Verification items for the finished model (mm, model axes). Face numbers are marked on the shaded views. A direction names the side the tool comes from. Give positions to 0.01 mm unless a question says otherwise; leave off trailing zeros. Order: outer loops, then holes, each group sorted by start corner. A loop starts at its lowest first (then second) coordinate and runs counter-clockwise, first axis right, second up.
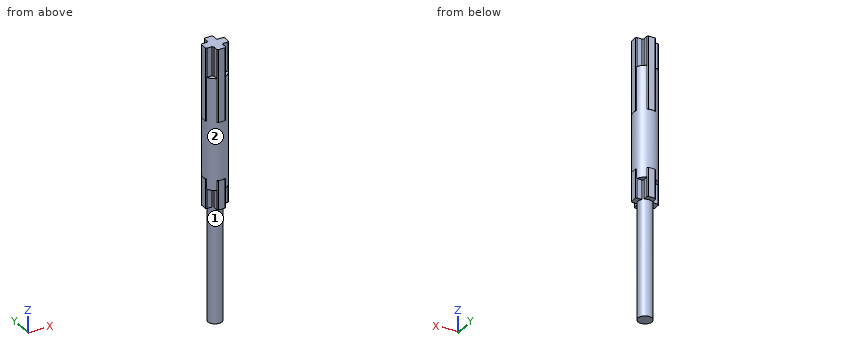
Autodesk Inventor part; units mm, degrees
ref_plane "Plano de trabajo1" through (0, -3.8636, 23) normal (0, 0, -1) x (-1, 0, 0)
ref_plane "Plano de trabajo2" through (0, 0, 0) normal (0, 0, 1) x (1, 0, 0)
ref_plane "YZ Plane" through (0, 0, 0) normal (1, 0, 0) x (0, 1, 0)
sketch "Boceto2" plane through (0, 0, 0) normal (0, 0, 1) x (1, 0, 0)
  line L0 (0.9, -6.2636) -> (-0.9, -6.2636)
  line L1 (-0.9, -6.2636) -> (-0.9, -1.4636)
  line L2 (-0.9, -1.4636) -> (0.9, -1.4636)
  line L3 (0.9, -1.4636) -> (0.9, -6.2636)
  line L4 (0.9, -6.2636) -> (-0.9, -1.4636) construction
  line L5 (-0.9, -6.2636) -> (0.9, -1.4636) construction
  line L6 (-2.4, -4.7636) -> (2.4, -4.7636)
  line L7 (2.4, -4.7636) -> (2.4, -2.9636)
  line L8 (2.4, -2.9636) -> (-2.4, -2.9636)
  line L9 (-2.4, -2.9636) -> (-2.4, -4.7636)
  line L10 (-2.4, -4.7636) -> (2.4, -2.9636) construction
  line L11 (2.4, -4.7636) -> (-2.4, -2.9636) construction
  circle A0 centre (0, -3.8636) radius 1.45
  point P0 (0, 0)
  point P1 (1.1369, -2.9636)
  point P2 (0.9, -2.7267)
  point P3 (-0.9, -2.7267)
  point P4 (-1.1369, -2.9636)
  point P5 (-1.1369, -4.7636)
  point P6 (-0.9, -5.0005)
  point P7 (0.9, -5.0005)
  point P8 (1.1369, -4.7636)
  dimension "d0" = 4.8
  dimension "d1" = 1.8
  dimension "d2" = 1.8
  dimension "d3" = 4.8
  dimension "d4" = 2.9
extrude "Extrusión1" add sketch "Boceto2" along normal blind 2 and the other way blind 4
sketch "Boceto3" plane through (0, 0, 2) normal (0, 0, 1) x (1, 0, 0)
  arc A0 (-0.9, -2.7267) -> (-1.1369, -2.9636) centre (0, -3.8636) ccw construction
  circle A1 centre (0, -3.8636) radius 1.45
  arc A2 (1.1369, -2.9636) -> (0.9, -2.7267) centre (0, -3.8636) ccw construction
  point P0 (0, 0)
  point P1 (1.0253, -2.8383)
extrude "Extrusión2" add sketch "Boceto3" along normal blind 12 and the other way blind 30
sketch "Boceto4" plane through (0, -3.8636, 14) normal (0, 0, 1) x (1, 0, 0)
  circle A0 centre (0, 0) radius 1.45 construction
  circle A1 centre (0, 0) radius 1.45
  line L0 (-0.9, 2.4) -> (0.9, 2.4) construction
  line L1 (0.9, -2.4) -> (-0.9, -2.4)
  line L2 (-0.9, -2.4) -> (-0.9, 2.4)
  line L3 (-0.9, 2.4) -> (0.9, 2.4)
  line L4 (0.9, 2.4) -> (0.9, -2.4)
  line L5 (0.9, -2.4) -> (-0.9, 2.4) construction
  line L6 (-0.9, -2.4) -> (0.9, 2.4) construction
  line L7 (2.4, 0.9) -> (-2.4, 0.9)
  line L8 (-2.4, 0.9) -> (-2.4, -0.9)
  line L9 (-2.4, -0.9) -> (2.4, -0.9)
  line L10 (2.4, -0.9) -> (2.4, 0.9)
  line L11 (2.4, 0.9) -> (-2.4, -0.9) construction
  line L12 (-2.4, 0.9) -> (2.4, -0.9) construction
  point P0 (1.1369, 0.9)
  point P1 (0.9, 1.1369)
  point P2 (-0.9, 1.1369)
  point P3 (-1.1369, 0.9)
  point P4 (-1.1369, -0.9)
  point P5 (-0.9, -1.1369)
  point P6 (0.9, -1.1369)
  point P7 (1.1369, -0.9)
extrude "Extrusión3" add sketch "Boceto4" along normal blind 15
chamfer "Chaflán1" distance 0.2 angle 45 16 edges at (0.9, -1.4636, -1) (-0.9, -1.4636, -1) (-2.4, -2.9636, -1) (-2.4, -4.7636, -1) (-0.9, -6.2636, -1) (0.9, -6.2636, -1) (2.4, -4.7636, -1) (2.4, -2.9636, -1) (2.4, -2.9636, 21.5) (0.9, -1.4636, 21.5) (-0.9, -1.4636, 21.5) (-2.4, -2.9636, 21.5) (-2.4, -4.7636, 21.5) (-0.9, -6.2636, 21.5) (0.9, -6.2636, 21.5) (2.4, -4.7636, 21.5)
ref_plane "Plano de trabajo1" through (0, -3.8636, 23) normal (0, 0, -1) x (-1, 0, 0)
sketch "Boceto5" plane through (0, -3.8636, 23) normal (0, 0, -1) x (-1, 0, 0)
  circle A0 centre (0, 0) radius 1.45 construction
  circle A1 centre (0, 0) radius 2.4
  line L0 (0.7, 2.4) -> (-0.7, 2.4) construction
  point P0 (0, 3.8636)
  point P1 (0, 2.4)
extrude "Extrusión4" add sketch "Boceto5" along normal blind 3
ref_plane "Plano de trabajo2" through (0, 0, 0) normal (0, 0, 1) x (1, 0, 0)
sketch "Boceto6" plane through (0, 0, 0) normal (0, 0, 1) x (1, 0, 0)
  arc A0 (-0.859, -1.6226) -> (-2.241, -3.0046) centre (0, -3.8636) ccw construction
  circle A1 centre (0, -3.8636) radius 2.4
  line L0 (0.7, -1.4636) -> (-0.7, -1.4636) construction
  point P0 (0, 0)
  point P1 (0, -1.4636)
extrude "Extrusión5" add sketch "Boceto6" along normal up to surface (20 mm away)
properties part number "EjeCilintroSuperiorGarra"
(1) Go/stop test with flat-tipped pins: pin 1 (1 mm diameter, centred on x = -2, y = -3.5, fed in from -Z); pin 2 (1.2 mm diameter, centred on y = -2, z = 25, fed in from -X); pin 3 (1.2 mm diameter, centred on y = -5.5, z = -1.5, fed in from -X). Record where each tip stops, or that it passes through.
Solved:
pin 1: stops at z = -4
pin 2: stops at x = -0.9
pin 3: stops at x = -1.01
(2) Section check A-A, the plane z = 16. Enter the section's corners in (x, y).
Solved:
outline: (-2.4, -4.56) - (-2.24, -4.72) arc R2.4 ccw to (-0.86, -6.1) - (-0.7, -6.26) - (0.7, -6.26) - (0.86, -6.1) arc R2.4 ccw to (2.24, -4.72) - (2.4, -4.56) - (2.4, -3.16) - (2.24, -3) arc R2.4 ccw to (0.86, -1.62) - (0.7, -1.46) - (-0.7, -1.46) - (-0.86, -1.62) arc R2.4 ccw to (-2.24, -3) - (-2.4, -3.16) - close
(3) Section check B-B, the plane z = -3. Enter the section's corners in (x, y).
Solved:
outline: (-2.4, -4.56) - (-2.2, -4.76) - (-1.14, -4.76) arc R1.45 ccw to (-0.9, -5) - (-0.9, -6.06) - (-0.7, -6.26) - (0.7, -6.26) - (0.9, -6.06) - (0.9, -5) arc R1.45 ccw to (1.14, -4.76) - (2.2, -4.76) - (2.4, -4.56) - (2.4, -3.16) - (2.2, -2.96) - (1.14, -2.96) arc R1.45 ccw to (0.9, -2.73) - (0.9, -1.66) - (0.7, -1.46) - (-0.7, -1.46) - (-0.9, -1.66) - (-0.9, -2.73) arc R1.45 ccw to (-1.14, -2.96) - (-2.2, -2.96) - (-2.4, -3.16) - close
(4) Set-up check for the marked faces 1 and 2: record each of +Z, -Z, +X, -X, +Y, -Y from which the full face is reachable in a straight line by a thin tool's end or side.
Solved:
face 1: -Z
face 2: none
(5) Scan lines: line 1 (Y direction, x = 2.25, z = 25.5); line 2 (Z direction, x = -1.2, y = -2.1); line 3 (Z direction, x = 0, y = -2.2). Record each from-to range of solid material in increasing order.
Solved:
line 1: y = -4.71 to -3.01
line 2: z = 0 to 23
line 3: z = -4 to 29
